For this review, use the dimensioned drawing (mm, ordinates from the lowest corner) and the shaded views. Round coordinates to 2 decimals unless told otherwise and drop trailing zeros. Write each loop counter-clockwise with the first axis right and the second up, starting at its lowest first coordinate (ties: lowest second). Pieces come first, ordered by that corner, then holes. Notation, with made-up numbers: (78, 66.25) -> (107, 66.25) arc R14 cw to (107, 73.25) -> close; hole circle Ø4 at (84.5, 54.25). An arc over 180 degrees is marked (long way). Answer in a Markdown table with one row per item. Add a question column.
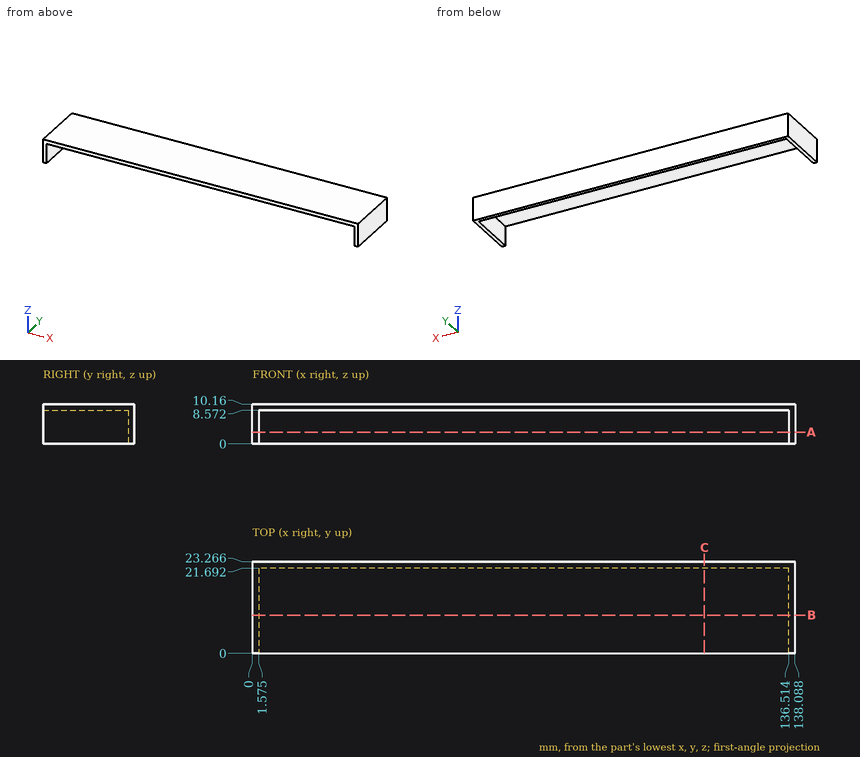
1. Clearance check with a flat-ended pin moving along its axis: pin 1 Ø5 at (x, y) = (120, 8) entering from -Z. State where the tip first meets the part, or that it passes through.
2. For L1, parallel to X at y = 3.75, z = 6 (1 decimal); L2, parallel to Z at x = 8.5, y = 3; L3, parallel to Y at x = 36.5, z = 2.25, list the stretches that pass through material, from the lowest coordinate up. Write a range as [from, to].
3. We need section B-B (y = 9.75). Write out the cut boundary in (x, z) (1 decimal).
4. We need section C-C (x = 115). Write out the cut boundary in (y, z).
5. We need section A-A (z = 3). Write out the cut boundary in (x, y) (1 decimal).
Response:
| question | item | result |
|---|---|---|
| 1 | pin 1 | z = 8.57 |
| 2 | L1 | [0, 1.6], [136.5, 138.1] |
| 2 | L2 | [8.57, 10.16] |
| 2 | L3 | [21.69, 23.27] |
| 3 | outline | (0, 0) -> (1.6, 0) -> (1.6, 8.6) -> (136.5, 8.6) -> (136.5, 0) -> (138.1, 0) -> (138.1, 10.2) -> (0, 10.2) -> close |
| 4 | outline | (0, 8.57) -> (21.69, 8.57) -> (21.69, 0) -> (23.27, 0) -> (23.27, 10.16) -> (0, 10.16) -> close |
| 5 | outline | (0, 0) -> (1.6, 0) -> (1.6, 21.7) -> (136.5, 21.7) -> (136.5, 0) -> (138.1, 0) -> (138.1, 23.3) -> (0, 23.3) -> close |
